from build123d import *

# Parameters (mm, degrees)
SKETCH1_W           = 11.7
SKETCH1_H           = 22.669491249
SKETCH1_W_2         = 3.4
SKETCH1_H_2         = 6.1
SKETCH1_R           = 1.475
SKETCH1_H_3         = 22.669491248
BOSS_EXTRUDE1_DEPTH = 5.58


with BuildPart() as part:
    # Sketch1 → Boss-Extrude1 (new body)
    with BuildSketch(Plane.XY):
        with BuildLine():
            Line((708.445729089, 432.610180658), (715.695729089, 432.610180658))
            Line((715.695729089, 432.610180658), (722.945729089, 432.610180658))
            ThreePointArc((722.945729089, 432.610180658), (726.481262995, 434.074646752), (727.945729089, 437.610180658))
            Line((727.945729089, 437.610180658), (727.945729089, 498.299163155))
            ThreePointArc((727.945729089, 498.299163155), (726.481262995, 501.834697061), (722.945729089, 503.299163155))
            Line((722.945729089, 503.299163155), (715.695729089, 503.299163155))
            Line((715.695729089, 503.299163155), (708.445729089, 503.299163155))
            ThreePointArc((708.445729089, 503.299163155), (704.910195183, 501.834697061), (703.445729089, 498.299163155))
            Line((703.445729089, 498.299163155), (703.445729089, 437.610180658))
            ThreePointArc((703.445729089, 437.610180658), (704.910195183, 434.074646752), (708.445729089, 432.610180658))
        make_face()
        with Locations((715.695729089, 448.944926283)):
            Rectangle(SKETCH1_W, SKETCH1_H, mode=Mode.SUBTRACT)
        with Locations((708.145729089, 463.429671907)):
            Rectangle(SKETCH1_W_2, SKETCH1_H_2, mode=Mode.SUBTRACT)
        with Locations((715.695729089, 467.954671907)):
            Circle(SKETCH1_R, mode=Mode.SUBTRACT)
        with Locations((723.245729089, 463.429671907)):
            Rectangle(SKETCH1_W_2, SKETCH1_H_2, mode=Mode.SUBTRACT)
        with Locations((708.145729089, 472.479671907)):
            Rectangle(SKETCH1_W_2, SKETCH1_H_2, mode=Mode.SUBTRACT)
        with Locations((715.695729089, 486.964417531)):
            Rectangle(SKETCH1_W, SKETCH1_H_3, mode=Mode.SUBTRACT)
        with Locations((723.245729089, 472.479671907)):
            Rectangle(SKETCH1_W_2, SKETCH1_H_2, mode=Mode.SUBTRACT)
    extrude(amount=BOSS_EXTRUDE1_DEPTH)


solid = part.part
Work out the finished part from the listing and answer in its coordinate system (mm). A direction names the side the tool comes from. Coordinates: 2 decimals unless noted, no trailing zeros. Loops run counter-clockwise (first coordinate to the right, second up) from the corner with the lowest first, then second, coordinate; pieces in that order, holes last. Notation, with made-up numbers: (76, 11) -> (112, 11) arc R9 ccw to (112, 17) -> close; hole circle Ø10 at (44.5, 68.25). An arc over 180 degrees is marked (long way). Write each question's results on one line, items separated by ' | '. Start each with the question number.
1) Find section B-B on x = 719.25. Determine the outline of the cut face in (y, z), then the cut area to 3 significant figures.
2) Find section C-C on z = 3.7. Count the separate pieces of the cut face and the enclosed holes in it, then the cut area to 3 significant figures.
3) Find section A-A on y = 453. Determine the outline of the cut face in (x, z).
4) Consider line 1 along X through (y, z) = (461.5, 4.6); line 2 along Y through (x, z) = (709, 2.55); line 3 along Y through (x, z) = (710.75, 2.45). Determine where each line is inside the solid, lowest interval first.
5) Find section D-D on x = 705.5. Determine the outline of the cut face in (y, z), then the cut area to 3 significant figures.
6) For faces 1 (the flat face through (718, 468, 5.58)), 2 (the flat face through (721.546, 487, 3)), determine the directions among +Z, -Z, +X, -X, +Y, -Y from which every point of the face is accessible in a straight line to the end or side of a thin tool.
Response values:
1) outline: (432.61, 0) -> (437.61, 0) -> (437.61, 5.58) -> (432.61, 5.58) -> close; (460.28, 0) -> (475.63, 0) -> (475.63, 5.58) -> (460.28, 5.58) -> close; (498.3, 0) -> (503.3, 0) -> (503.3, 5.58) -> (498.3, 5.58) -> close | area: 141 mm^2
2) separate pieces: 1 | enclosed holes: 7 | area: 1,090 mm^2
3) outline: (703.45, 0) -> (709.85, 0) -> (709.85, 5.58) -> (703.45, 5.58) -> close; (721.55, 0) -> (727.95, 0) -> (727.95, 5.58) -> (721.55, 5.58) -> close
4) line 1: x = 703.45 to 706.45, 709.85 to 721.55, 724.95 to 727.95 | line 2: y = 432.61 to 460.38, 466.48 to 469.43, 475.53 to 503.3 | line 3: y = 432.61 to 437.61, 460.28 to 475.63, 498.3 to 503.3
5) outline: (433.57, 0) -> (502.34, 0) -> (502.34, 5.58) -> (433.57, 5.58) -> close | area: 384 mm^2
6) face 1: +Z, +X, -X, +Y, -Y | face 2: +Z, -Z
